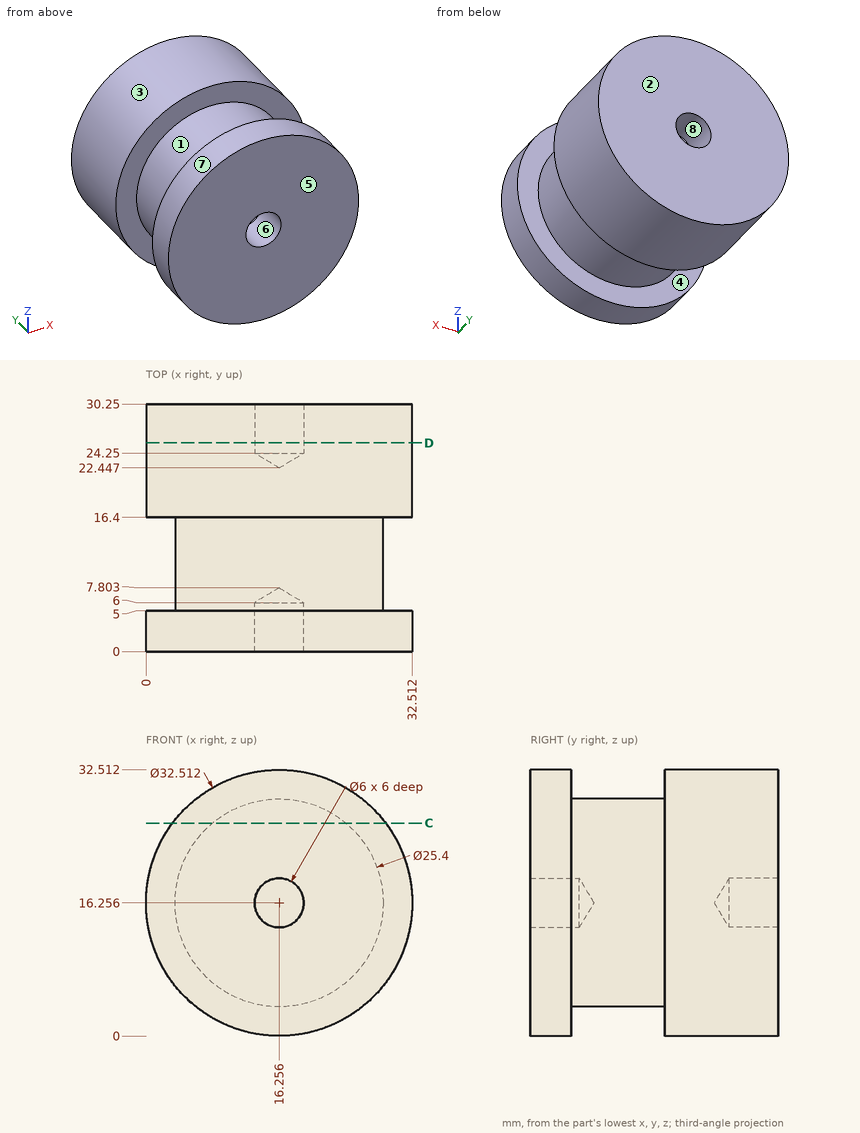
Part print with two shaded views. Sizes in mm from the minimum x, y, z corner. A direction names the side the tool comes from. Round coordinates to 2 decimals unless told otherwise and drop trailing zeros. Loops run counter-clockwise (first coordinate to the right, second up) from the corner with the lowest first, then second, coordinate; pieces in that order, holes last. Notation, with made-up numbers: M -22,32.5 L 34,32.5 A14 cw 34,57.5 Z; hole C 41,-12 d4. An arc over 180 degrees is marked long. Return JSON: item names as keys, results as strings. Group by question number.
(1) Saw through at D-D, the plane y = 25.5. List the corners of the cut face in (x, z), and give its area (3 significant figures).
(2) Drop flat-ended pins along their axis: P1, Ø8, axis at x = 19.5, y = 21.5, coming from the -Z side; P2, Ø10, axis at x = 3.5, y = 18.5, coming from the +Z side; P3, Ø3, axis at y = 21.5, z = 12, coming from the -X side (1 decimal); P4, Ø4, axis at x = 28, y = 22.5, coming from the +Z side. Give the stop position or say it passes through.
(3) Saw through at C-C, the plane z = 26. List the corners of the cut face in (x, y).
(4) Wall check: probe 1 along Y at (x, z) = (29, 15); probe 2 along X at (y, z) = (29.5, 14) (1 decimal); probe 3 along Z at (x, y) = (22, 19). Give the ranges that are in metal, low to high. Write a range as [from, to].
(5) Mould opens along Y. For the marked faces 1, 2 and 3 say: +Y half, -Y half, draft (parallel to the pull), parting line (faces both ways), or undercut.
(6) Tool access for the marked faces 4, 5, 6, 7 and 8: list every direction of +Z, -Z, +X, -X, +Y, -Y with a clear straight run to the whole face (end or side of a thin tool).
Answer list:
{
 "1": {"outline": "C 16.26,16.26 d32.51; hole C 16.26,16.26 d6", "area": "802 mm2"},
 "2": {"P1": "z = 0", "P2": "z = 30.54", "P3": "x = 0.2", "P4": "z = 29.27"},
 "3": {"outline": "M 3.24,0 L 29.27,0 L 29.27,5 L 24.4,5 L 24.4,16.4 L 29.27,16.4 L 29.27,30.25 L 3.24,30.25 L 3.24,16.4 L 8.11,16.4 L 8.11,5 L 3.24,5 Z"},
 "4": {"probe 1": "[0, 5], [16.4, 30.25]", "probe 2": "[0.2, 14.3], [18.2, 32.4]", "probe 3": "[1.05, 31.46]"},
 "5": {"face 1": "undercut", "face 2": "+Y half", "face 3": "draft"},
 "6": {"face 4": "none", "face 5": "+Z, -Z, +X, -X, -Y", "face 6": "-Y", "face 7": "+Y, -Y", "face 8": "+Y"}
}
